from build123d import *

# Parameters (mm, degrees)
F0_R     = 7.5
F1_DEPTH = 25
F2_R     = 10
F3_DEPTH = 15
F4_R     = 15
F5_DEPTH = 10
F6_R     = 12.5
F7_DEPTH = 10


with BuildPart() as f1:
    # F0 (on Front) → F1 (new body)
    with BuildSketch(Plane.XZ):
        Circle(F0_R)
    extrude(amount=F1_DEPTH)

    # F2 (on face) → F3 (join)
    with BuildSketch(Plane(origin=(0, 0, 0), x_dir=(-1, 0, 0), z_dir=(0, 1, 0))):
        Circle(F2_R)
    extrude(amount=F3_DEPTH)

    # F4 (on face) → F5 (join)
    with BuildSketch(Plane(origin=(0, 15, 0), x_dir=(-1, 0, 0), z_dir=(0, 1, 0))):
        Circle(F4_R)
    extrude(amount=F5_DEPTH)

    # F6 (on face) → F7 (join)
    with BuildSketch(Plane(origin=(0, 25, 0), x_dir=(-1, 0, 0), z_dir=(0, 1, 0))):
        Circle(F6_R)
    extrude(amount=F7_DEPTH)


solid = f1.part
Could you check a few things on this model? Use its own coordinates, in mm. A direction names the side the tool comes from. Coordinates: 2 decimals unless noted, no trailing zeros. Order: outer loops, then holes, each group sorted by start corner. A loop starts at its lowest first (then second) coordinate and runs counter-clockwise, first axis right, second up.
Q1. Which directions (+Z, -Z, +X, -X, +Y, -Y) give clear straight access to the entire face, cutting with the end or side of a thin tool? Please do faces 1 (the flat face through (0, -25, 0)), 2 (the cylindrical face through (2.17, 7.4, -9.76)), 3 (the flat face through (3.4, 25, 12.3)).
Q2. Suppose I cut it at C-C on y = -15.5. Please give me the cut outline in (x, z), and give its area (3 significant figures).
Q3. Suppose I cut it at A-A on z = 0. Please give me the cut outline in (x, y), and give its area (4 significant figures).
Q4. Suppose I cut it at B-B on x = 0. Please give me the cut outline in (y, z).
Q5. Will these pins go through, and if not, where does the flat tip stop? pin 1 (1.5 mm diameter, centred on y = -0.5, z = -8.5, fed in from +X); pin 2 (5 mm diameter, centred on x = -0.5, y = -6, fed in from -Z); pin 3 (8 mm diameter, centred on x = -6, z = -11.5, fed in from -Y); pin 4 (10 mm diameter, centred on x = 1.5, y = 18, fed in from +Z).
Q6. Please list where these lines run through material, in increasing order: L1, parallel to Y at x = 5, z = -12.25; L2, parallel to Y at x = -4.75, z = 10.5; L3, parallel to Z at x = -6.5, y = 25.5.
Answer:
1. face 1: +Z, -Z, +X, -X, -Y
1. face 2: -Y
1. face 3: +Y
2. outline: circle Ø15 at (0, 0)
2. area: 177 mm2
3. outline: (-15, 15) - (-10, 15) - (-10, 0) - (-7.5, 0) - (-7.5, -25) - (7.5, -25) - (7.5, 0) - (10, 0) - (10, 15) - (15, 15) - (15, 25) - (12.5, 25) - (12.5, 35) - (-12.5, 35) - (-12.5, 25) - (-15, 25) - close
3. area: 1,225 mm2
4. outline: (-25, -7.5) - (0, -7.5) - (0, -10) - (15, -10) - (15, -15) - (25, -15) - (25, -12.5) - (35, -12.5) - (35, 12.5) - (25, 12.5) - (25, 15) - (15, 15) - (15, 10) - (0, 10) - (0, 7.5) - (-25, 7.5) - close
5. pin 1: stops at x = 6.08
5. pin 2: stops at z = -7.5
5. pin 3: stops at y = 0
5. pin 4: stops at z = 15
6. L1: y = 15 to 25
6. L2: y = 15 to 35
6. L3: z = -10.68 to 10.68
